Job drawing, mm, ordinate dimensions from the low corner. One solid piece. Round coordinates to 2 decimals unless told otherwise and drop trailing zeros. Order: outer loops, then holes, each group sorted by start corner. A loop starts at its lowest first (then second) coordinate and runs counter-clockwise, first axis right, second up. Notation, with made-up numbers: M 6.25,32 L 30.25,32 A31 cw 30.25,68 Z; hole C 7,32 d2. An arc over 180 degrees is marked long. Answer as a JSON object with one key per item and string values. Group by question number.
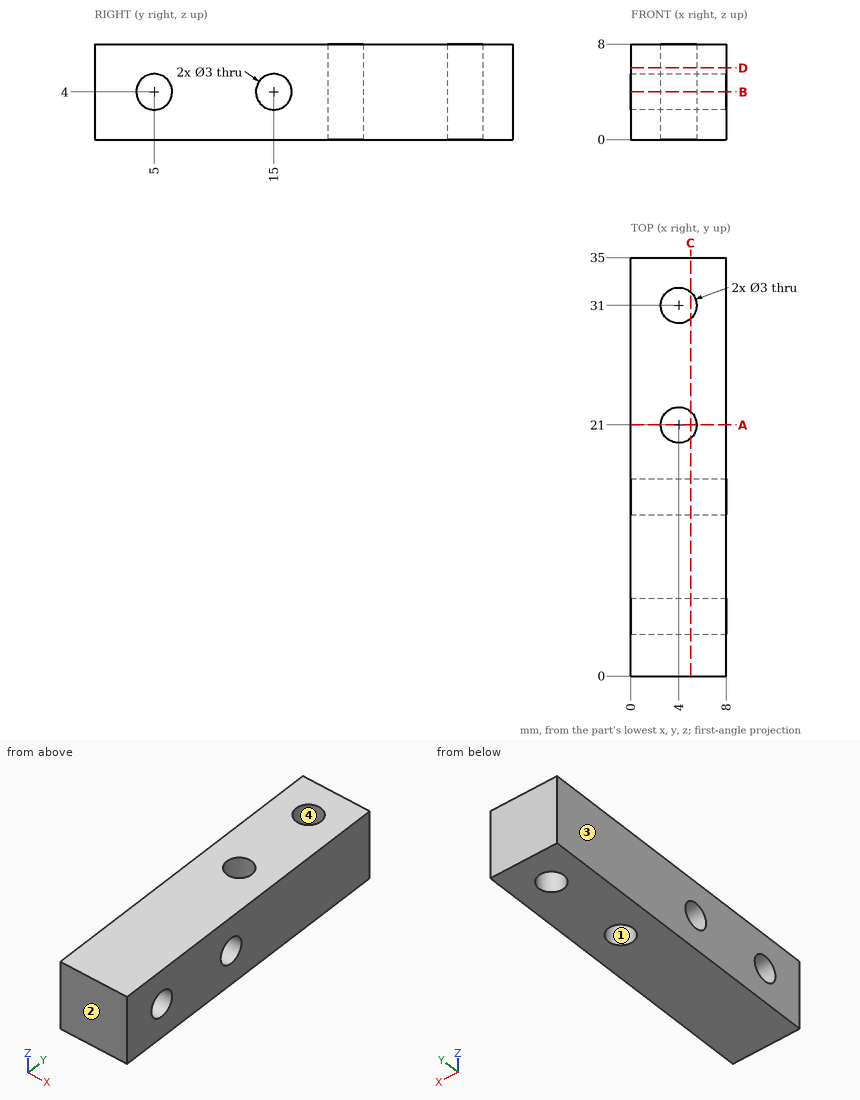
Item 1: Cut at B-B, the plane z = 4. Give the cut face in (x, y), and give its area (3 significant figures).
Item 2: Two-plate mould, pull along Y, no slides. Class the marked faces 1, 2, 3 and 4: +Y half, -Y half, draft (parallel to the pull), parting line (faces both ways), or undercut.
Item 3: Cut at C-C, the plane x = 5. Give the cut face in (y, z).
Item 4: Cut at D-D, the plane z = 6. Give the cut face in (x, y).
Item 5: Drill centre lines: line 1 (Y direction, x = 6, z = 4); line 2 (Y direction, x = 4, z = 3.75); line 3 (Y direction, x = 6, z = 5). Where is each one in solid material? Low to high. Write a range as [from, to].
Item 6: Cut at A-A, the plane y = 21. Give the cut face in (x, z).
Response values:
{
 "1": {"outline": "M 0,0 L 8,0 L 8,3.5 L 0,3.5 Z; M 0,6.5 L 8,6.5 L 8,13.5 L 0,13.5 Z; M 0,16.5 L 8,16.5 L 8,35 L 0,35 Z; hole C 4,21 d3; hole C 4,31 d3", "area": "218 mm^2"},
 "2": {"face 1": "undercut", "face 2": "-Y half", "face 3": "draft", "face 4": "undercut"},
 "3": {"outline": "M 0,0 L 19.88,0 L 19.88,8 L 0,8 Z; M 22.12,0 L 29.88,0 L 29.88,8 L 22.12,8 Z; M 32.12,0 L 35,0 L 35,8 L 32.12,8 Z; hole C 5,4 d3; hole C 15,4 d3"},
 "4": {"outline": "M 0,0 L 8,0 L 8,35 L 0,35 Z; hole C 4,21 d3; hole C 4,31 d3"},
 "5": {"line 1": "[0, 3.5], [6.5, 13.5], [16.5, 35]", "line 2": "[0, 3.52], [6.48, 13.52], [16.48, 19.5], [22.5, 29.5], [32.5, 35]", "line 3": "[0, 3.88], [6.12, 13.88], [16.12, 35]"},
 "6": {"outline": "M 0,0 L 2.5,0 L 2.5,8 L 0,8 Z; M 5.5,0 L 8,0 L 8,8 L 5.5,8 Z"}
}
